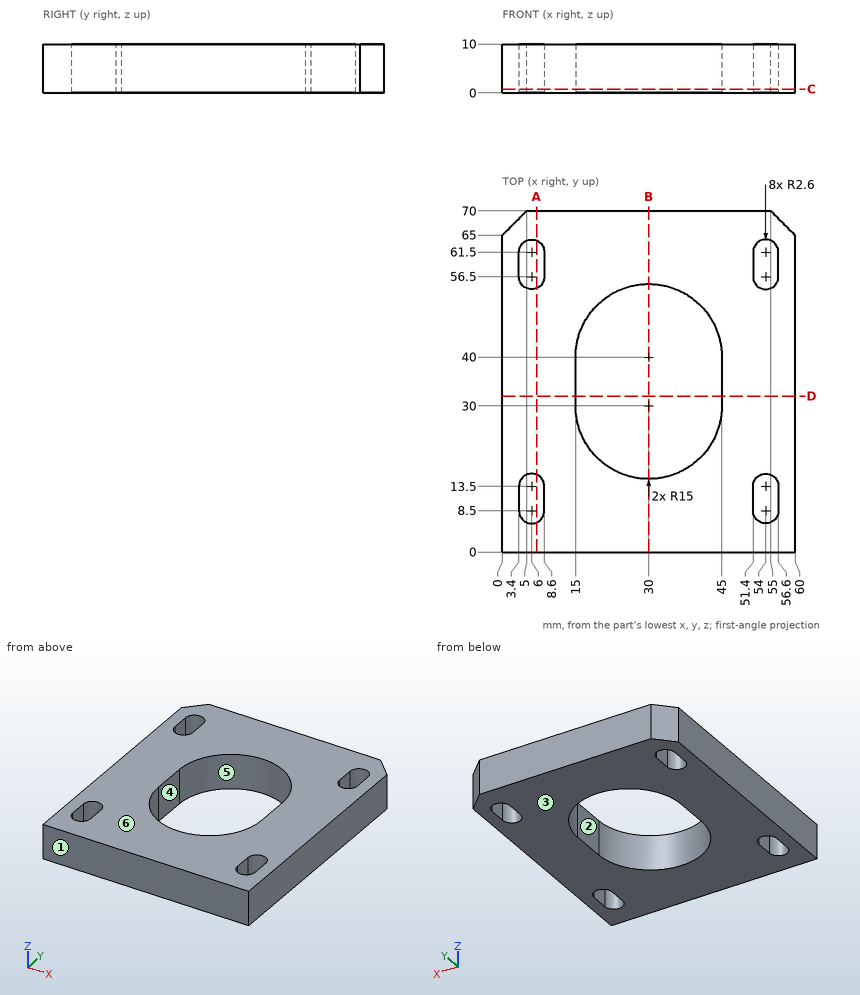
For this review, use the dimensioned drawing (mm, ordinates from the lowest corner) and the shaded views. A direction names the side the tool comes from. Round coordinates to 2 decimals unless told otherwise and drop trailing zeros. Order: outer loops, then holes, each group sorted by start corner. A loop starts at its lowest first (then second) coordinate and runs counter-clockwise, first axis right, second up. Notation, with made-up numbers: (67.5, -3.5) - (112.5, -3.5) arc R25 ccw to (112.5, 10.5) - close; hole circle Ø1 at (18, 41.25). An arc over 180 degrees is marked (long way). Use one line per item in the form item = value.
Q1. Add section C-C on z = 0.75. Give the boundary of the cut face in (x, y).
Response values:
outline = (0, 0) - (60, 0) - (60, 65) - (55, 70) - (5, 70) - (0, 65) - close; hole (3.4, 8.5) arc R2.6 ccw to (8.6, 8.5) - (8.6, 13.5) arc R2.6 ccw to (3.4, 13.5) - close; hole (3.4, 56.5) arc R2.6 ccw to (8.6, 56.5) - (8.6, 61.5) arc R2.6 ccw to (3.4, 61.5) - close; hole (15, 30) arc R15 ccw to (45, 30) - (45, 40) arc R15 ccw to (15, 40) - close; hole (51.4, 8.5) arc R2.6 ccw to (56.6, 8.5) - (56.6, 13.5) arc R2.6 ccw to (51.4, 13.5) - close; hole (51.4, 56.5) arc R2.6 ccw to (56.6, 56.5) - (56.6, 61.5) arc R2.6 ccw to (51.4, 61.5) - close
Q2. Tool access review of the marked faces 5 and 6: name each direction out of +Z, -Z, +X, -X, +Y, -Y from which nothing blocks a thin tool from reaching the whole face with its end or side.
Response values:
face_5 = +Z, -Z
face_6 = +Z, +X, -X, +Y, -Y
Q3. Add section D-D on y = 32. Give the boundary of the cut face in (x, z), then the cut area to 3 significant figures.
Response values:
outline = (0, 0) - (15, 0) - (15, 10) - (0, 10) - close; (45, 0) - (60, 0) - (60, 10) - (45, 10) - close
area = 300 mm^2
Q4. Add section B-B on x = 30. Give the boundary of the cut face in (y, z).
Response values:
outline = (0, 0) - (15, 0) - (15, 10) - (0, 10) - close; (55, 0) - (70, 0) - (70, 10) - (55, 10) - close
Q5. Add section A-A on x = 7. Give the boundary of the cut face in (y, z), then the cut area to 3 significant figures.
Response values:
outline = (0, 0) - (6.1, 0) - (6.1, 10) - (0, 10) - close; (15.9, 0) - (54.1, 0) - (54.1, 10) - (15.9, 10) - close; (63.9, 0) - (70, 0) - (70, 10) - (63.9, 10) - close
area = 504 mm^2
Q6. Mouldability with a two-part tool opening along Y and no side actions: class the marked faces 1, 2, 3 and 4 as pulls with the +Y half, pulls with the -Y half, needs draft (parallel to the pull), parting line crosses it, or undercut.
Response values:
face_1 = pulls with the -Y half
face_2 = undercut
face_3 = needs draft
face_4 = undercut
Q7. To check wall thickness, follow line 1 (X direction, y = 12, z = 1.5); line 2 (Y direction, x = 6, z = 7.75); line 3 (X direction, y = 40.5, z = 2.5). State the ranges of each line that lie inside material, in increasing order.
Response values:
line_1 = 0 to 3.4, 8.6 to 51.4, 56.6 to 60
line_2 = 0 to 5.9, 16.1 to 53.9, 64.1 to 70
line_3 = 0 to 15.01, 44.99 to 60
